from build123d import *

# Parameters (mm, degrees)
BOSS_EXTRUDE1_DEPTH = 110.3


with BuildPart() as part:
    # Sketch1 → Boss-Extrude1 (new body)
    with BuildSketch(Plane(origin=(0, 0, 0), x_dir=(1, 0, 0), z_dir=(0, 1, 0))):
        with BuildLine():
            Line((-8, 8), (-4.949747468, 4.949747468))
            ThreePointArc((-4.949747468, 4.949747468), (2.678784027, 6.467156728), (7, 0))
            ThreePointArc((7, 0), (6.467156728, -2.678784027), (4.949747468, -4.949747468))
            Line((4.949747468, -4.949747468), (8, -8))
            ThreePointArc((8, -8), (10.197365132, -4.900382063), (11.244655102, -1.248091194))
            ThreePointArc((11.244655102, -1.248091194), (10.063708499, 0), (11.244655102, 1.248091194))
            ThreePointArc((11.244655102, 1.248091194), (8, 8), (1.248091194, 11.244655102))
            ThreePointArc((1.248091194, 11.244655102), (0, 10.063708499), (-1.248091194, 11.244655102))
            ThreePointArc((-1.248091194, 11.244655102), (-4.900382063, 10.197365132), (-8, 8))
        make_face()
        with BuildLine():
            Line((-11.313708499, 11.313708499), (-8, 8))
            ThreePointArc((-8, 8), (-4.900382063, 10.197365132), (-1.248091194, 11.244655102))
            ThreePointArc((-1.248091194, 11.244655102), (-0.034539887, 12.563231206), (1.25, 11.313708499))
            ThreePointArc((1.25, 11.313708499), (1.249522707, 11.279168612), (1.248091194, 11.244655102))
            ThreePointArc((1.248091194, 11.244655102), (8, 8), (11.244655102, 1.248091194))
            ThreePointArc((11.244655102, 1.248091194), (12.17283109, 0.907969368), (12.563708499, 0))
            ThreePointArc((12.563708499, 0), (12.17283109, -0.907969368), (11.244655102, -1.248091194))
            ThreePointArc((11.244655102, -1.248091194), (10.197365132, -4.900382063), (8, -8))
            Line((8, -8), (11.313708499, -11.313708499))
            ThreePointArc((11.313708499, -11.313708499), (14.78207252, -6.122934918), (16, 0))
            ThreePointArc((16, 0), (6.122934918, 14.78207252), (-11.313708499, 11.313708499))
        make_face()
    extrude(amount=BOSS_EXTRUDE1_DEPTH)


solid = part.part
Work out the finished part from the listing and answer in its coordinate system (mm). Round coordinates to 2 decimals unless told otherwise and drop trailing zeros. Write each loop counter-clockwise with the first axis right and the second up, starting at its lowest first coordinate (ties: lowest second). Pieces come first, ordered by that corner, then holes. Notation, with made-up numbers: M -27,21.25 L -13,21.25 A32 ccw -13,57.25 Z; hole C 72,4 d11. An arc over 180 degrees is marked long. Use a Markdown table: item, result.
1) The part is cut by section C-C on z = -3.5. Give the vertices of the cut face in (x, y).
Taken from the geometry:
| item | result |
|---|---|
| outline | M 6.06,0 L 15.61,0 L 15.61,110.3 L 6.06,110.3 Z |
2) The part is cut by section D-D on x = -8.75. Give the vertices of the cut face in (y, z).
Taken from the geometry:
| item | result |
|---|---|
| outline | M 0,-13.4 L 110.3,-13.4 L 110.3,-8.75 L 0,-8.75 Z |
3) Flat-ended cylindrical pins translate along their axes: pin 1 (6 mm diameter, centred on x = 6, y = 65, fed in from +Z); pin 2 (4 mm diameter, centred on x = 10, y = 75.5, fed in from +Z); pin 3 (3 mm diameter, centred on x = -7.5, y = 59.5, fed in from +Z). Find the tip coordinate at first contact, or state that the pin passes through.
Taken from the geometry:
| item | result |
|---|---|
| pin 1 | stops at z = 9 |
| pin 2 | stops at z = 11.31 |
| pin 3 | stops at z = -6 |
4) The part is cut by section A-A on x = 0. Give the vertices of the cut face in (y, z).
Taken from the geometry:
| item | result |
|---|---|
| outline | M 0,-16 L 110.3,-16 L 110.3,-12.56 L 0,-12.56 Z; M 0,-10.06 L 110.3,-10.06 L 110.3,-7 L 0,-7 Z |
5) Consider line 1 (Z direction, x = 11.75, y = 25); line 2 (X direction, y = 99.5, z = 0.5); line 3 (Z direction, x = 10.25, y = 78.5). Determine where each line is inside the solid, lowest interval first. Write a range as [from, to].
Taken from the geometry:
| item | result |
|---|---|
| line 1 | z = [-10.86, -1.17], [1.17, 10.86] |
| line 2 | x = [6.98, 10.17], [12.46, 15.99] |
| line 3 | z = [-12.29, -0.66], [0.66, 10.25] |
